The listing builds one solid part. Answer for the finished solid, in the listing's coordinates (mm). A direction names the side the tool comes from. Coordinates: 2 decimals unless noted, no trailing zeros. Loops run counter-clockwise (first coordinate to the right, second up) from the corner with the lowest first, then second, coordinate; pieces in that order, holes last. Notation, with made-up numbers: (6, 18) -> (48, 18) arc R24 cw to (48, 32) -> close; hole circle Ø8 at (37.5, 2). An arc over 180 degrees is marked (long way). Answer in a Markdown table with one row per item.
```python
from build123d import *

# Parameters (mm, degrees)
SKETCH1_W           = 50.8
SKETCH1_H           = 25.4
SKETCH1_W_2         = 44.45
SKETCH1_H_2         = 19.05
BOSS_EXTRUDE1_DEPTH = 457.2
SKETCH2_R           = 2.5
CUT_EXTRUDE1_DEPTH  = 459.608940166


with BuildPart() as part:
    # Sketch1 → Boss-Extrude1 (new body)
    with BuildSketch(Plane(origin=(0, 0, 0), x_dir=(1, 0, 0), z_dir=(0, 1, 0))):
        Rectangle(SKETCH1_W, SKETCH1_H)
        Rectangle(SKETCH1_W_2, SKETCH1_H_2, mode=Mode.SUBTRACT)
    extrude(amount=BOSS_EXTRUDE1_DEPTH)

    # Sketch2 → Cut-Extrude1 (cut, through all)
    with BuildSketch(Plane.XY.offset(12.7)):
        with Locations((-11.25, 60)):
            Circle(SKETCH2_R)
        with Locations((-11.25, 25)):
            Circle(SKETCH2_R)
        with Locations((11.25, 25)):
            Circle(SKETCH2_R)
        with Locations((11.25, 60)):
            Circle(SKETCH2_R)
    extrude(amount=-CUT_EXTRUDE1_DEPTH, mode=Mode.SUBTRACT)


solid = part.part
```
Item 1: A flat-ended cylindrical pin translates along its axis: pin 1 Ø3 at (x, y) = (11.25, 25) entering from +Z. Find the tip coordinate at first contact, or state that the pin passes through.
Findings below:
| item | result |
|---|---|
| pin 1 | passes through |
Item 2: A cutting plane is placed at B-B, the plane x = -1. Determine the outline of the cut face in (y, z) (3 decimals).
Findings below:
| item | result |
|---|---|
| outline | (0, -12.7) -> (457.2, -12.7) -> (457.2, -9.525) -> (0, -9.525) -> close; (0, 9.525) -> (457.2, 9.525) -> (457.2, 12.7) -> (0, 12.7) -> close |
Item 3: Determine the mould class of faces 1 (the face through (25.4, 225, 0)), 2 (the face through (0, 457.2, -10)), 3 (the face through (-25.4, 225, 0)), 4 (the face through (0, 225, 9.525)) for opening direction X: +X half, -X half, draft (parallel to the pull), parting line (faces both ways), or undercut.
Findings below:
| item | result |
|---|---|
| face 1 | +X half |
| face 2 | draft |
| face 3 | -X half |
| face 4 | undercut |
Item 4: Find the intervals of material crossed by probe 1 along Y at (x, z) = (-11.25, -10.3); probe 2 along Z at (x, y) = (17, 43) (3 decimals); probe 3 along X at (y, z) = (372.5, 2) (3 decimals), in increasing order.
Findings below:
| item | result |
|---|---|
| probe 1 | y = 0 to 22.5, 27.5 to 57.5, 62.5 to 457.2 |
| probe 2 | z = -12.7 to -9.525, 9.525 to 12.7 |
| probe 3 | x = -25.4 to -22.225, 22.225 to 25.4 |
Item 5: A cutting plane is placed at A-A, the plane z = -3.5. Determine the outline of the cut face in (x, y) (3 decimals), plus the area to 3 significant figures.
Findings below:
| item | result |
|---|---|
| outline | (-25.4, 0) -> (-22.225, 0) -> (-22.225, 457.2) -> (-25.4, 457.2) -> close; (22.225, 0) -> (25.4, 0) -> (25.4, 457.2) -> (22.225, 457.2) -> close |
| area | 2,900 mm2 |
Item 6: A tool of negligible diameter and unlimited length cuts with its end or side. For faces 5 (the face through (0, 225, -12.7)), 6 (the face through (22.225, 225, 0)), from which of +Z, -Z, +X, -X, +Y, -Y can it reach the whole face along a straight path? Write none if from no direction.
Findings below:
| item | result |
|---|---|
| face 5 | -Z, +X, -X, +Y, -Y |
| face 6 | +Y, -Y |
Item 7: A cutting plane is placed at C-C, the plane y = 414. Determine the outline of the cut face in (x, z) (3 decimals), plus the area to 3 significant figures.
Findings below:
| item | result |
|---|---|
| outline | (-25.4, -12.7) -> (25.4, -12.7) -> (25.4, 12.7) -> (-25.4, 12.7) -> close; hole (-22.225, -9.525) -> (22.225, -9.525) -> (22.225, 9.525) -> (-22.225, 9.525) -> close |
| area | 444 mm2 |
